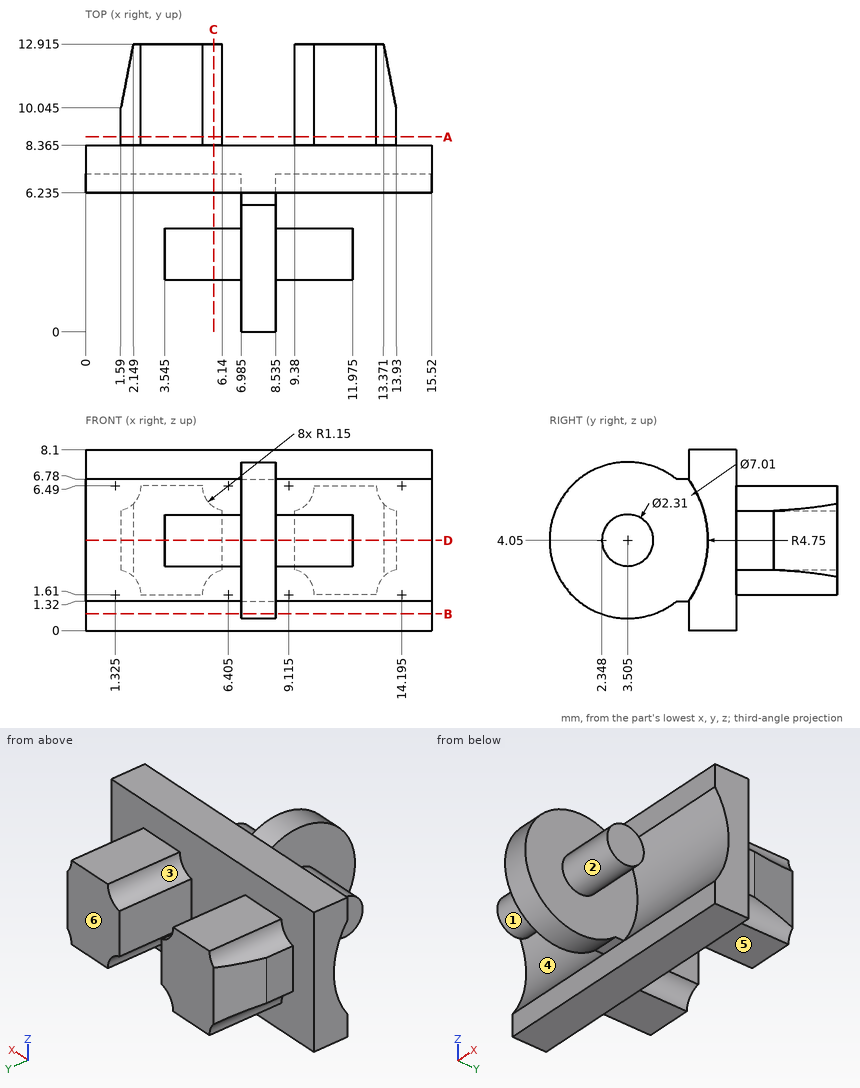
Geometry: see drawing. Coordinates: mm, zero at the bounding-box minimum. A direction names the side the tool comes from. Coordinates: 2 decimals unless noted, no trailing zeros. Loops run counter-clockwise (first coordinate to the right, second up) from the corner with the lowest first, then second, coordinate; pieces in that order, holes last. Notation, with made-up numbers: M 7,34.25 L 34,34.25 A19 cw 34,46.25 Z; hole C 89.5,41.5 d8. An arc over 180 degrees is marked long. Put each result on its own line as item: value. Start each with the question number.
1) Pull-direction query (Y, two-part tool) for the marked faces 4, 5 and 6; classes: pulls with the +Y half, pulls with the -Y half, needs draft (parallel to the pull), parting line crosses it, or undercut.
2) Contact query for flat-ended pins moving along their axis: pin 1 Ø0.7 at (x, z) = (7.5, 7.5) entering from -Y; pin 2 Ø1 at (y, z) = (2.5, 4) entering from +X (3 decimals); pin 3 Ø3 at (x, y) = (11, 9.5) entering from +Z; pin 4 Ø1.5 at (y, z) = (4.5, 7) entering from +X (3 decimals). Output: stop coordinate, or through.
3) Cut plane B-B on z = 0.75. Return the cut outline in (x, y) (3 decimals), then the cut area to 3 significant figures.
4) Cut plane D-D on z = 4.05. Return the cut outline in (x, y) (3 decimals).
5) Cut plane A-A on y = 8.75. Return the cut outline in (x, z) (3 decimals).
6) Reachability of the marked faces 1, 2 and 3 from +Z, -Z, +X, -X, +Y, -Y: full face, straight path, thin tool, end or side. Return the list, or none.
7) Ray query, L1, parallel to Y at x = 5, z = 0.5 (3 decimals); L2, parallel to Y at x = 11.75, z = 3.25 (1 decimal); L3, parallel to X at y = 1, z = 5.25 (3 decimals). Return the intervals inside material, ascending. Write a range as from..to.
8) Cut plane C-C on x = 5.75. Return the cut outline in (y, z) (3 decimals).
The answers:
1. face 4: undercut
1. face 5: needs draft
1. face 6: pulls with the +Y half
2. pin 1: stops at y = 1.87
2. pin 2: stops at x = 11.975
2. pin 3: stops at z = 8.1
2. pin 4: stops at x = 8.535
3. outline: M 0,6.235 L 15.52,6.235 L 15.52,8.365 L 0,8.365 Z; M 6.985,2.324 L 8.535,2.324 L 8.535,4.686 L 6.985,4.686 Z
3. area: 36.7 mm²
4. outline: M 0,7.098 L 6.985,7.098 L 6.985,4.66 L 3.545,4.66 L 3.545,2.35 L 6.985,2.35 L 6.985,0 L 8.535,0 L 8.535,2.35 L 11.975,2.35 L 11.975,4.66 L 8.535,4.66 L 8.535,7.098 L 15.52,7.098 L 15.52,8.365 L 13.93,8.365 L 13.93,10.045 L 13.371,12.915 L 9.38,12.915 L 9.38,8.365 L 6.14,8.365 L 6.14,12.915 L 2.149,12.915 L 1.59,10.045 L 1.59,8.365 L 0,8.365 Z
5. outline: M 1.59,2.729 A1.15 cw 2.475,1.61 L 5.255,1.61 A1.15 cw 6.14,2.729 L 6.14,5.371 A1.15 cw 5.255,6.49 L 2.475,6.49 A1.15 cw 1.59,5.371 Z; M 9.38,2.729 A1.15 cw 10.265,1.61 L 13.045,1.61 A1.15 cw 13.93,2.729 L 13.93,5.371 A1.15 cw 13.045,6.49 L 10.265,6.49 A1.15 cw 9.38,5.371 Z
6. face 1: -X
6. face 2: +X
6. face 3: +Z, +Y
7. L1: y = 6.235..8.365
7. L2: y = 2.7..4.3, 7..12.9
7. L3: x = 6.985..8.535
8. outline: C 3.505,4.05 d2.31; M 6.235,0 L 8.365,0 L 8.365,2.555 L 12.915,2.555 L 12.915,5.545 L 8.365,5.545 L 8.365,8.1 L 6.235,8.1 L 6.235,6.78 A4.75 cw 6.235,1.32 Z
